Design review of the part shown in the three views and the two pictorial views. Dimensions are in mm from the part's minimum x, y and z. A direction names the side the tool comes from. Round coordinates to 2 decimals unless told otherwise and drop trailing zeros. Write each loop counter-clockwise with the first axis right and the second up, starting at its lowest first coordinate (ties: lowest second). Pieces come first, ordered by that corner, then holes. Notation, with made-up numbers: (79, -4) - (97, -4) arc R20 cw to (97, 15) - close; hole circle Ø8 at (84, -28). An arc over 180 degrees is marked (long way). Use one line per item in the form item = value.
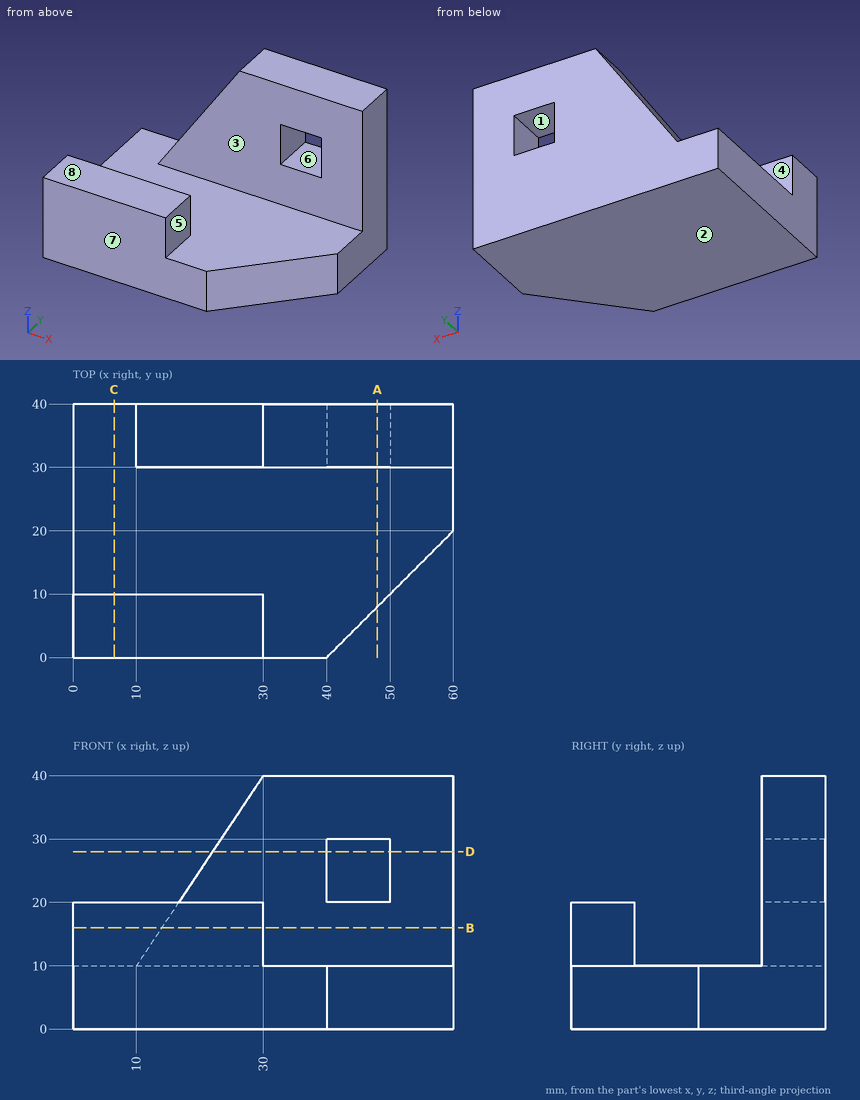
(1) Machinability: for the marked faces 4, 5, 6, 7 and 8, which of the approach directions +Z, -Z, +X, -X, +Y, -Y give a long, thin tool a straight path to every point of the face, cutting with its end or side? Answer none if there is none.
Geometry results:
face_4 = +Z, +X, -X
face_5 = +Z, +X, -Y
face_6 = +Y, -Y
face_7 = +Z, -Z, +X, -X, -Y
face_8 = +Z, +X, -X, -Y
(2) Add section C-C on x = 6.5. Write out the cut boundary in (y, z).
Geometry results:
outline = (0, 0) - (40, 0) - (40, 10) - (10, 10) - (10, 20) - (0, 20) - close
(3) Add section D-D on z = 28. Write out the cut boundary in (x, y).
Geometry results:
outline = (22, 30) - (40, 30) - (40, 40) - (22, 40) - close; (50, 30) - (60, 30) - (60, 40) - (50, 40) - close
(4) To check wall thickness, follow L1, parallel to Y at x = 21, z = 15; L2, parallel to Y at x = 32.5, z = 37; L3, parallel to Z at x = 24.5, y = 25. State the ranges of each line that lie inside material, in increasing order.
Geometry results:
L1 = 0 to 10, 30 to 40
L2 = 30 to 40
L3 = 0 to 10
(5) The part is to be moulded in two halves that separate along Z. For the marked faces 1, 2 and 3, say which applies: +Z half, -Z half, draft (parallel to the pull), parting line (faces both ways), or undercut.
Geometry results:
face_1 = undercut
face_2 = -Z half
face_3 = draft
(6) Add section A-A on x = 48. Write out the cut boundary in (y, z), then the cut area to 3 significant figures.
Geometry results:
outline = (8, 0) - (40, 0) - (40, 20) - (30, 20) - (30, 10) - (8, 10) - close; (30, 30) - (40, 30) - (40, 40) - (30, 40) - close
area = 520 mm2
(7) Add section B-B on z = 16. Write out the cut boundary in (x, y), then the cut area to 3 significant figures.
Geometry results:
outline = (0, 0) - (30, 0) - (30, 10) - (0, 10) - close; (14, 30) - (60, 30) - (60, 40) - (14, 40) - close
area = 760 mm2
(8) Insertion check: P1, Ø11, axis at x = 8, y = 3.5, coming from the +Z side; P2, Ø6, axis at y = 25, z = 30.5, coming from the +X side; P3, Ø24, axis at x = 33.5, z = 32, coming from the -Y side; P4, Ø1.5, axis at x = 10.5, y = 26, coming from the +Z side. Each pin has a flat end and moves straight along its axis. Give the tip position at first contact, or say it passes through.
Geometry results:
P1 = 20
P2 = through
P3 = 30
P4 = 10
